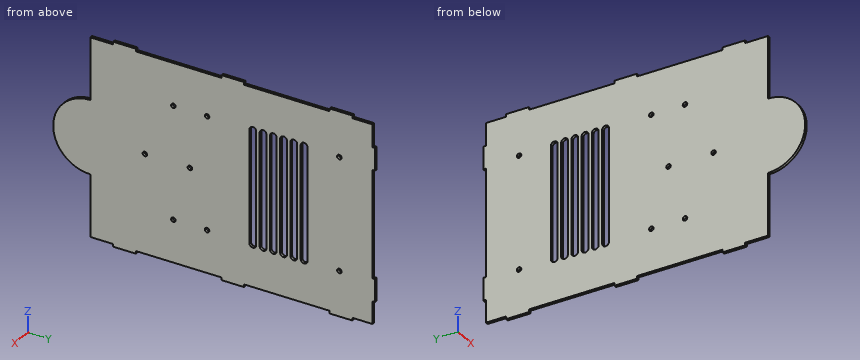
from build123d import *

# Parameters (mm, degrees)
BOSS_EXTRUDE1_DEPTH = 2.3622
SKETCH2_R           = 2
CUT_EXTRUDE1_DEPTH  = 242.723455562


with BuildPart() as part:
    # Sketch1 → Boss-Extrude1 (new body)
    with BuildSketch(Plane(origin=(0, 0, 0), x_dir=(0, 0, -1), z_dir=(1, 0, 0))):
        with BuildLine():
            Line((-130.13293856, 199.80032679), (-130.13293856, 182.16252679))
            Line((-130.13293856, 182.16252679), (-132.49513856, 182.16252679))
            Line((-132.49513856, 182.16252679), (-132.49513856, 162.16252679))
            Line((-132.49513856, 162.16252679), (-130.13293856, 162.16252679))
            Line((-130.13293856, 162.16252679), (-130.13293856, 87.16252679))
            Line((-130.13293856, 87.16252679), (-132.49513856, 87.16252679))
            Line((-132.49513856, 87.16252679), (-132.49513856, 67.16252679))
            Line((-132.49513856, 67.16252679), (-130.13293856, 67.16252679))
            Line((-130.13293856, 67.16252679), (-130.13293856, -7.83747321))
            Line((-130.13293856, -7.83747321), (-132.49513856, -7.83747321))
            Line((-132.49513856, -7.83747321), (-132.49513856, -27.83747321))
            Line((-132.49513856, -27.83747321), (-130.13293856, -27.83747321))
            Line((-130.13293856, -27.83747321), (-130.13293856, -47.83747321))
            Line((-130.13293856, -47.83747321), (-75.13293856, -47.83747321))
            ThreePointArc((-75.13293856, -47.83747321), (-42.49513856, -80.47527321), (-9.85733856, -47.83747321))
            Line((-9.85733856, -47.83747321), (45.14266144, -47.83747321))
            Line((45.14266144, -47.83747321), (45.14266144, -27.83747321))
            Line((45.14266144, -27.83747321), (47.50486144, -27.83747321))
            Line((47.50486144, -27.83747321), (47.50486144, -7.83747321))
            Line((47.50486144, -7.83747321), (45.14266144, -7.83747321))
            Line((45.14266144, -7.83747321), (45.14266144, 67.16252679))
            Line((45.14266144, 67.16252679), (47.50486144, 67.16252679))
            Line((47.50486144, 67.16252679), (47.50486144, 87.16252679))
            Line((47.50486144, 87.16252679), (45.14266144, 87.16252679))
            Line((45.14266144, 87.16252679), (45.14266144, 162.16252679))
            Line((45.14266144, 162.16252679), (47.50486144, 162.16252679))
            Line((47.50486144, 162.16252679), (47.50486144, 182.16252679))
            Line((47.50486144, 182.16252679), (45.14266144, 182.16252679))
            Line((45.14266144, 182.16252679), (45.14266144, 199.80032679))
            Line((45.14266144, 199.80032679), (25.14266144, 199.80032679))
            Line((25.14266144, 199.80032679), (25.14266144, 202.16252679))
            Line((25.14266144, 202.16252679), (5.14266144, 202.16252679))
            Line((5.14266144, 202.16252679), (5.14266144, 199.80032679))
            Line((5.14266144, 199.80032679), (-90.13293856, 199.80032679))
            Line((-90.13293856, 199.80032679), (-90.13293856, 202.16252679))
            Line((-90.13293856, 202.16252679), (-110.13293856, 202.16252679))
            Line((-110.13293856, 202.16252679), (-110.13293856, 199.80032679))
            Line((-110.13293856, 199.80032679), (-130.13293856, 199.80032679))
        make_face()
    extrude(amount=BOSS_EXTRUDE1_DEPTH)

    # Sketch2 → Cut-Extrude1 (cut, through all)
    with BuildSketch(Plane(origin=(2.3622, 0, 0), x_dir=(0, 0, -1), z_dir=(1, 0, 0))):
        with Locations((-92.49513856, 54.59655139)):
            Circle(SKETCH2_R)
        with Locations((7.50486144, 54.59655139)):
            Circle(SKETCH2_R)
        with Locations((7.50486144, 25.043037435)):
            Circle(SKETCH2_R)
        with Locations((-92.49513856, 170.771110124)):
            Circle(SKETCH2_R)
        with Locations((7.50486144, 170.771110124)):
            Circle(SKETCH2_R)
        with Locations((-92.49513856, 25.043037435)):
            Circle(SKETCH2_R)
        with Locations((-42.49513856, 39.546662347)):
            Circle(SKETCH2_R)
        with Locations((-42.49513856, 0)):
            Circle(SKETCH2_R)
        with BuildLine():
            Line((-92.49513856, 142.80032679), (7.50486144, 142.80032679))
            ThreePointArc((7.50486144, 142.80032679), (10.50486144, 139.80032679), (7.50486144, 136.80032679))
            Line((7.50486144, 136.80032679), (-92.49513856, 136.80032679))
            ThreePointArc((-92.49513856, 136.80032679), (-95.49513856, 139.80032679), (-92.49513856, 142.80032679))
        make_face()
        with BuildLine():
            Line((-92.49513856, 133.80032679), (7.50486144, 133.80032679))
            ThreePointArc((7.50486144, 133.80032679), (10.50486144, 130.80032679), (7.50486144, 127.80032679))
            Line((7.50486144, 127.80032679), (-92.49513856, 127.80032679))
            ThreePointArc((-92.49513856, 127.80032679), (-95.49513856, 130.80032679), (-92.49513856, 133.80032679))
        make_face()
        with BuildLine():
            Line((-92.49513856, 124.80032679), (7.50486144, 124.80032679))
            ThreePointArc((7.50486144, 124.80032679), (10.50486144, 121.80032679), (7.50486144, 118.80032679))
            Line((7.50486144, 118.80032679), (-92.49513856, 118.80032679))
            ThreePointArc((-92.49513856, 118.80032679), (-95.49513856, 121.80032679), (-92.49513856, 124.80032679))
        make_face()
        with BuildLine():
            Line((-92.49513856, 115.80032679), (7.50486144, 115.80032679))
            ThreePointArc((7.50486144, 115.80032679), (10.50486144, 112.80032679), (7.50486144, 109.80032679))
            Line((7.50486144, 109.80032679), (-92.49513856, 109.80032679))
            ThreePointArc((-92.49513856, 109.80032679), (-95.49513856, 112.80032679), (-92.49513856, 115.80032679))
        make_face()
        with BuildLine():
            Line((-92.49513856, 106.80032679), (7.50486144, 106.80032679))
            ThreePointArc((7.50486144, 106.80032679), (10.50486144, 103.80032679), (7.50486144, 100.80032679))
            Line((7.50486144, 100.80032679), (-92.49513856, 100.80032679))
            ThreePointArc((-92.49513856, 100.80032679), (-95.49513856, 103.80032679), (-92.49513856, 106.80032679))
        make_face()
        with BuildLine():
            Line((-92.49513856, 97.80032679), (7.50486144, 97.80032679))
            ThreePointArc((7.50486144, 97.80032679), (10.50486144, 94.80032679), (7.50486144, 91.80032679))
            Line((7.50486144, 91.80032679), (-92.49513856, 91.80032679))
            ThreePointArc((-92.49513856, 91.80032679), (-95.49513856, 94.80032679), (-92.49513856, 97.80032679))
        make_face()
    extrude(amount=-CUT_EXTRUDE1_DEPTH, mode=Mode.SUBTRACT)


solid = part.part
Geometry: final body of the model. Coordinates: model frame, mm. Coordinates: 2 decimals unless noted, no trailing zeros. Order: outer loops, then holes, each group sorted by start corner. A loop starts at its lowest first (then second) coordinate and runs counter-clockwise, first axis right, second up.
(1) First-contact query: pin 1 (0.7 mm diameter, centred on x = 1.5, z = 131, fed in from +Y); pin 2 (1.2 mm diameter, centred on x = 1, z = 65, fed in from +Y); pin 3 (1.2 mm diameter, centred on x = 1.5, z = 62.5, fed in from -Y). Flat tips, straight axial feed; report the tip coordinate or a pass-through.
(2) Material intervals for probe 1 along Z at (x, y) = (1.45, 113); probe 2 along Z at (x, y) = (0.3, 40); probe 3 along Z at (x, y) = (1.55, 184), sorted ascending.
(3) Section query D-D (x = 1.85). State how many separate pieces and enclosed holes the cut face has, plus the area to 3 significant figures.
(4) Section query B-B (y = -31.5). Return the cut outline in (x, z), plus the area to 3 significant figures.
(5) Section query A-A (z = 85.5). Return the cut outline in (x, y), plus the area to 3 significant figures.
(6) Section query C-C (z = 62). Return the cut outline in (x, y).
Solution:
1. pin 1: stops at y = 182.16
1. pin 2: stops at y = 199.8
1. pin 3: stops at y = -74.08
2. probe 1: z = -45.14 to -10.5, 95.49 to 130.13
2. probe 2: z = -45.14 to 40.55, 44.44 to 130.13
2. probe 3: z = -45.14 to 130.13
3. separate pieces: 1
3. enclosed holes: 14
3. area: 41,600 mm2
4. outline: (0, -45.14) - (2.36, -45.14) - (2.36, 130.13) - (0, 130.13) - close
4. area: 414 mm2
5. outline: (0, -47.84) - (2.36, -47.84) - (2.36, 91.8) - (0, 91.8) - close; (0, 97.8) - (2.36, 97.8) - (2.36, 100.8) - (0, 100.8) - close; (0, 106.8) - (2.36, 106.8) - (2.36, 109.8) - (0, 109.8) - close; (0, 115.8) - (2.36, 115.8) - (2.36, 118.8) - (0, 118.8) - close; (0, 124.8) - (2.36, 124.8) - (2.36, 127.8) - (0, 127.8) - close; (0, 133.8) - (2.36, 133.8) - (2.36, 136.8) - (0, 136.8) - close; (0, 142.8) - (2.36, 142.8) - (2.36, 199.8) - (0, 199.8) - close
5. area: 500 mm2
6. outline: (0, -74.01) - (2.36, -74.01) - (2.36, 91.8) - (0, 91.8) - close; (0, 97.8) - (2.36, 97.8) - (2.36, 100.8) - (0, 100.8) - close; (0, 106.8) - (2.36, 106.8) - (2.36, 109.8) - (0, 109.8) - close; (0, 115.8) - (2.36, 115.8) - (2.36, 118.8) - (0, 118.8) - close; (0, 124.8) - (2.36, 124.8) - (2.36, 127.8) - (0, 127.8) - close; (0, 133.8) - (2.36, 133.8) - (2.36, 136.8) - (0, 136.8) - close; (0, 142.8) - (2.36, 142.8) - (2.36, 199.8) - (0, 199.8) - close
